```python
from build123d import *

# Parameters (mm, degrees)
F0_W = 50.8
F0_H = 41.3327284643
F4_T = 2.286


# Not quite as in the source:
# - the arcs of a loft's sections are written as splines that run evenly, so that the points pair up as in the source's solid
# - a shell that OpenCascade refuses in one call is made with other operations: the cavity is built on its own and cut out


with BuildPart() as f3:
    # F0 (on Top) → F3 section 0
    with BuildSketch(Plane.XY):
        Rectangle(F0_W, F0_H)
    # F2 (on offset) → F3 section 1
    with BuildSketch(Plane.XY.offset(50.8)):
        with BuildLine():
            add(Edge.make_bspline(
                [(16.0305352967, 13.0430268219), (15.1768711874, 14.0922229036), (14.2198939474, 15.0573165448), (12.135995559, 16.7823054792), (11.0091259391, 17.5421581187), (8.6287404272, 18.8274534668), (7.3752833949, 19.3528643939), (4.7898876398, 20.1490729763), (3.458012846, 20.4198509437), (0.7669621567, 20.696374911), (-0.5921471973, 20.7021140733), (-3.2854372521, 20.4483267645), (-4.6195513559, 20.1888065689), (-7.2115791497, 19.414460888), (-8.4694287466, 18.8996545501), (-10.8605841049, 17.6345081674), (-11.9938307403, 16.8841994059), (-13.0430268219, 16.0305352967)],
                knots=[0, 0, 0, 0, 0.125, 0.125, 0.25, 0.25, 0.375, 0.375, 0.5, 0.5, 0.625, 0.625, 0.75, 0.75, 0.875, 0.875, 1, 1, 1, 1], degree=3))
            add(Edge.make_bspline(
                [(-13.0430268219, 16.0305352967), (-14.0922229036, 15.1768711874), (-15.0573165448, 14.2198939474), (-16.7823054792, 12.135995559), (-17.5421581187, 11.0091259391), (-18.8274534668, 8.6287404272), (-19.3528643939, 7.3752833949), (-20.1490729763, 4.7898876398), (-20.4198509437, 3.458012846), (-20.696374911, 0.7669621567), (-20.7021140733, -0.5921471973), (-20.4483267645, -3.2854372521), (-20.1888065689, -4.6195513559), (-19.414460888, -7.2115791497), (-18.8996545501, -8.4694287466), (-17.6345081674, -10.8605841049), (-16.8841994059, -11.9938307403), (-16.0305352967, -13.0430268219)],
                knots=[0, 0, 0, 0, 0.125, 0.125, 0.25, 0.25, 0.375, 0.375, 0.5, 0.5, 0.625, 0.625, 0.75, 0.75, 0.875, 0.875, 1, 1, 1, 1], degree=3))
            add(Edge.make_bspline(
                [(-16.0305352967, -13.0430268219), (-15.1768711874, -14.0922229036), (-14.2198939474, -15.0573165448), (-12.135995559, -16.7823054792), (-11.0091259391, -17.5421581187), (-8.6287404272, -18.8274534668), (-7.3752833949, -19.3528643939), (-4.7898876398, -20.1490729763), (-3.458012846, -20.4198509437), (-0.7669621567, -20.696374911), (0.5921471973, -20.7021140733), (3.2854372521, -20.4483267645), (4.6195513559, -20.1888065689), (7.2115791497, -19.414460888), (8.4694287466, -18.8996545501), (10.8605841049, -17.6345081674), (11.9938307403, -16.8841994059), (13.0430268219, -16.0305352967)],
                knots=[0, 0, 0, 0, 0.125, 0.125, 0.25, 0.25, 0.375, 0.375, 0.5, 0.5, 0.625, 0.625, 0.75, 0.75, 0.875, 0.875, 1, 1, 1, 1], degree=3))
            add(Edge.make_bspline(
                [(13.0430268219, -16.0305352967), (14.0922229036, -15.1768711874), (15.0573165448, -14.2198939474), (16.7823054792, -12.135995559), (17.5421581187, -11.0091259391), (18.8274534668, -8.6287404272), (19.3528643939, -7.3752833949), (20.1490729763, -4.7898876398), (20.4198509437, -3.458012846), (20.696374911, -0.7669621567), (20.7021140733, 0.5921471973), (20.4483267645, 3.2854372521), (20.1888065689, 4.6195513559), (19.414460888, 7.2115791497), (18.8996545501, 8.4694287466), (17.6345081674, 10.8605841049), (16.8841994059, 11.9938307403), (16.0305352967, 13.0430268219)],
                knots=[0, 0, 0, 0, 0.125, 0.125, 0.25, 0.25, 0.375, 0.375, 0.5, 0.5, 0.625, 0.625, 0.75, 0.75, 0.875, 0.875, 1, 1, 1, 1], degree=3))
        make_face()
    loft(ruled=True)

    # F4: shell of thickness 2.286, made by hand


with BuildPart() as f4_core1:
    # F4_t2: copy of F3
    add(f3.part)

    # the walls: a layer under each face that stays
    f4_faces = [f4_core1.faces().sort_by_distance(p)[0] for p in [
        (22.9790564637, -1.0562437507, 25.4),
        (1.0562437507, 20.6122385797, 25.4),
        (-22.9790564637, 1.0562437507, 25.4),
        (-1.0562437507, -20.6122385797, 25.4),
        (0, 0, 50.8),
    ]]
    thicken(f4_faces, amount=-F4_T, mode=Mode.SUBTRACT)


with BuildPart() as f3_1:
    add(f3.part)

    # what is left inside the walls is the cavity
    f4_cavity = [f4_core1.part.solids().sort_by_distance(p)[0] for p in [
        (-0.625568, -18.323309, 16.343336),
    ]]
    add(f4_cavity, mode=Mode.SUBTRACT)


solid = f3_1.part
```
Model file for the job. Use its own axes, mm. Give positions to 0.01 mm unless a question says otherwise; leave off trailing zeros. Write each question's results on one line, items separated by ' | '.
(1) Flat gauge pins, fed straight in: pin 1 Ø3 at (x, z) = (-20, 16.5) entering from +Y; pin 2 Ø10 at (x, y) = (-4, 5) entering from -Z; pin 3 Ø4 at (y, z) = (10, 14.5) entering from -X; pin 4 Ø12 at (x, y) = (19.5, 15) entering from -Z. Where does each tip first touch, or does it go through?
Geometry results:
pin 1: stops at y = 19.62 | pin 2: stops at z = 48.51 | pin 3: stops at x = -23.7 | pin 4: stops at z = 0
(2) Pull direction X, two halves, no side cores. Call faces 1 (the flat face through (0, 0, 50.8)), 2 (the flat face through (0, 0, 48.514)): released by +X, released by -X, zero draft, split by the parting line, or undercut.
Geometry results:
face 1: zero draft | face 2: undercut
(3) Probe line 1 along Z through (x, y) = (2, 14); line 2 along Y through (x, z) = (11, 6); line 3 along Y through (x, z) = (16.5, 29.5). List the from-to ranges inside material, lowest first.
Geometry results:
line 1: z = 48.51 to 50.8 | line 2: y = -20.58 to -18.3, 18.13 to 20.42 | line 3: y = -18.51 to -16.1, 15.15 to 17.61
